Design review of the part built by this model. Coordinates are the model's own, in mm. A direction names the side the tool comes from. Round coordinates to 2 decimals unless told otherwise and drop trailing zeros. Write each loop counter-clockwise with the first axis right and the second up, starting at its lowest first coordinate (ties: lowest second). Pieces come first, ordered by that corner, then holes. Notation, with made-up numbers: (71, -34.75) - (123, -34.75) arc R20 cw to (123, -27.75) - close; hole circle Ø10 at (37, 70). An arc over 180 degrees is marked (long way). Use one line per item in the form item = value.
```python
from build123d import *

# Parameters (mm, degrees)
SKETCH1_W               = 26
SKETCH1_H               = 40
BOSS_EXTRUDE1_DEPTH     = 32
SKETCH2_W               = 21
SKETCH2_H               = 34.5
CUT_EXTRUDE1_DEPTH      = 28
SKETCH3_W               = 26
SKETCH3_H               = 25.26
BOSS_EXTRUDE2_DEPTH     = 20
SKETCH4_W               = 22
SKETCH4_H               = 19.76
CUT_EXTRUDE2_DEPTH      = 20
SKETCH5_W               = 21
SKETCH5_H               = 2.75
CUT_EXTRUDE3_DEPTH      = 25
SKETCH6_R               = 1.1
CUT_EXTRUDE4_DEPTH      = 20
SKETCH7_R               = 4
CUT_EXTRUDE5_DEPTH      = 5
SKETCH9_W               = 26
SKETCH9_H               = 25.26
CUT_EXTRUDE9_DEPTH      = 3
SKETCH10_R              = 4.8
SKETCH10_R_2            = 4
BOSS_EXTRUDE3_DEPTH     = 3
CUT_EXTRUDE10_DEPTH     = 5
SKETCH14_W              = 1.5
SKETCH14_H              = 19.76
BOSS_EXTRUDE5_DEPTH     = 17
SKETCH8_R               = 1
SKETCH8_R_2             = 1.3
CUT_EXTRUDE8_DEPTH      = 17
CUT_EXTRUDE8_DEPTH_BACK = 15
SKETCH17_W              = 26
SKETCH17_H              = 25.26
SKETCH17_W_2            = 20.5
SKETCH17_H_2            = 19.76
BOSS_EXTRUDE12_DEPTH    = 12
SKETCH18_W              = 21
SKETCH18_H              = 12
CUT_EXTRUDE11_DEPTH     = 5


with BuildPart() as part:
    # Sketch1 → Boss-Extrude1 (new body)
    with BuildSketch(Plane.XY):
        with Locations((-13, 20)):
            Rectangle(SKETCH1_W, SKETCH1_H)
    extrude(amount=BOSS_EXTRUDE1_DEPTH)

    # Sketch2 → Cut-Extrude1 (cut)
    with BuildSketch(Plane.XY.offset(32)):
        with Locations((-13, 20)):
            Rectangle(SKETCH2_W, SKETCH2_H)
    extrude(amount=-CUT_EXTRUDE1_DEPTH, mode=Mode.SUBTRACT)

    # Sketch3 → Boss-Extrude2 (add)
    with BuildSketch(Plane.XY.offset(32)):
        with Locations((-13, 12.63)):
            Rectangle(SKETCH3_W, SKETCH3_H)
    extrude(amount=BOSS_EXTRUDE2_DEPTH)

    # Sketch4 → Cut-Extrude2 (cut)
    with BuildSketch(Plane.XY.offset(52)):
        with Locations((-13, 12.63)):
            Rectangle(SKETCH4_W, SKETCH4_H)
    extrude(amount=-CUT_EXTRUDE2_DEPTH, mode=Mode.SUBTRACT)

    # Sketch5 → Cut-Extrude3 (cut)
    with BuildSketch(Plane.XY.offset(32)):
        with Locations((-13, 38.625)):
            Rectangle(SKETCH5_W, SKETCH5_H)
    extrude(amount=-CUT_EXTRUDE3_DEPTH, mode=Mode.SUBTRACT)

    # Sketch6 → Cut-Extrude4 (cut)
    with BuildSketch(Plane(origin=(0, 0, 0), x_dir=(-1, 0, 0), z_dir=(0, 0, -1))):
        with Locations((4.8, 4.55)):
            Circle(SKETCH6_R)
        with Locations((20.8, 4.55)):
            Circle(SKETCH6_R)
        with Locations((20.8, 34.55)):
            Circle(SKETCH6_R)
        with Locations((4.8, 34.55)):
            Circle(SKETCH6_R)
    extrude(amount=-CUT_EXTRUDE4_DEPTH, mode=Mode.SUBTRACT)

    # Sketch7 → Cut-Extrude5 (cut)
    with BuildSketch(Plane.ZY.offset(26)):
        with Locations((40, 12.51)):
            Circle(SKETCH7_R)
    extrude(amount=-CUT_EXTRUDE5_DEPTH, mode=Mode.SUBTRACT)

    # Sketch9 → Cut-Extrude9 (cut)
    with BuildSketch(Plane.XY.offset(52)):
        with Locations((-13, 12.63)):
            Rectangle(SKETCH9_W, SKETCH9_H)
    extrude(amount=-CUT_EXTRUDE9_DEPTH, mode=Mode.SUBTRACT)

    # Sketch10 → Boss-Extrude3 (add)
    with BuildSketch(Plane.ZY.offset(26)):
        with Locations((40, 12.51)):
            Circle(SKETCH10_R)
        with Locations((40, 12.51)):
            Circle(SKETCH10_R_2, mode=Mode.SUBTRACT)
    extrude(amount=BOSS_EXTRUDE3_DEPTH)

    # Sketch13 → Cut-Extrude10 (cut, through all)
    with BuildSketch(Plane.XY.offset(4)):
        Polygon((-23.5, 20), (-23.5, 12), (-2.5, 12), (-2.5, 29), (-23.5, 29), align=None)
    extrude(amount=-CUT_EXTRUDE10_DEPTH, mode=Mode.SUBTRACT)

    # Sketch14 → Boss-Extrude5 (add)
    with BuildSketch(Plane.XY.offset(49)):
        with Locations((-2.75, 12.63)):
            Rectangle(SKETCH14_W, SKETCH14_H)
    extrude(amount=-BOSS_EXTRUDE5_DEPTH)

    # Sketch8 → Cut-Extrude8 (cut, two sides)
    with BuildSketch(Plane(origin=(0, 0, 0), x_dir=(0, 0, -1), z_dir=(1, 0, 0))) as cut_extrude8_sk:
        with Locations((-40, 12.51)):
            Circle(SKETCH8_R)
        with Locations((-46, 12.51)):
            Circle(SKETCH8_R_2)
        with Locations((-34, 12.51)):
            Circle(SKETCH8_R_2)
        with Locations((-40, 18.51)):
            Circle(SKETCH8_R_2)
        with Locations((-40, 6.51)):
            Circle(SKETCH8_R_2)
    extrude(amount=CUT_EXTRUDE8_DEPTH, mode=Mode.SUBTRACT)
    extrude(cut_extrude8_sk.sketch, amount=-CUT_EXTRUDE8_DEPTH_BACK, mode=Mode.SUBTRACT)

    # Sketch17 → Boss-Extrude12 (add)
    with BuildSketch(Plane.XY.offset(49)):
        with Locations((-13, 12.63)):
            Rectangle(SKETCH17_W, SKETCH17_H)
        with Locations((-13.75, 12.63)):
            Rectangle(SKETCH17_W_2, SKETCH17_H_2, mode=Mode.SUBTRACT)
    extrude(amount=BOSS_EXTRUDE12_DEPTH)

    # Sketch18 → Cut-Extrude11 (cut)
    with BuildSketch(Plane(origin=(0, 25.26, 0), x_dir=(1, 0, 0), z_dir=(0, 1, 0))):
        with Locations((-13, -38)):
            Rectangle(SKETCH18_W, SKETCH18_H)
    extrude(amount=-CUT_EXTRUDE11_DEPTH, mode=Mode.SUBTRACT)


solid = part.part
```
Q1. Machinability: for faces 4 (the flat face through (0, 15, 30)), 5 (the flat face through (-1, 33, 32)), 6 (the cylindrical face through (-1.73, 6.57, 41.3)), 7 (the flat face through (-13, 33, 4)), 8 (the flat face through (-13, 40, 5)), which of the approach directions +Z, -Z, +X, -X, +Y, -Y give a long, thin tool a straight path to every point of the face, cutting with its end or side? Answer none if there is none.
Calculated:
face_4 = +Z, -Z, +X, +Y, -Y
face_5 = +Z, +X, -X, +Y
face_6 = +X
face_7 = +Z
face_8 = +Z, -Z, +X, -X, +Y
Q2. We need section C-C on x = -9. Write out the cut boundary in (y, z).
Calculated:
outline = (0, 0) - (12, 0) - (12, 4) - (2.75, 4) - (2.75, 61) - (0, 61) - close; (22.51, 44) - (25.26, 44) - (25.26, 61) - (22.51, 61) - close; (29, 0) - (40, 0) - (40, 7) - (37.25, 7) - (37.25, 4) - (29, 4) - close
Q3. For P1, Ø5, axis at x = -25.5, z = 27, coming from the -Y side; P2, Ø9, axis at x = -12.5, y = 34.5, coming from the +Z side; P3, Ø2.5, axis at y = 12.51, z = 40, coming from the -X side; P4, Ø3, axis at x = -19, y = 4.5, coming from the +Z side, all flat-tipped, find the tip position at first contact; note any pin that passes through.
Calculated:
P1 = 0
P2 = 7
P3 = -3.5
P4 = 4
Q4. To check wall thickness, follow line 1 along Y through (x, z) = (-20.8, 1); line 2 along X through (y, z) = (5, 20.5); line 3 along X through (y, z) = (15, 45). State the ranges of each line that lie inside material, in increasing order. Write a range as from..to.
Calculated:
line_1 = 0..3.45, 5.65..12, 29..33.45, 35.65..40
line_2 = -26..-23.5, -2.5..0
line_3 = -26..-24, -3.5..0
Q5. We need section A-A on y = 34.55. Write out the cut boundary in (x, z), then the cut area to 3 significant figures.
Calculated:
outline = (-26, 0) - (-21.9, 0) - (-21.9, 4) - (-23.5, 4) - (-23.5, 32) - (-26, 32) - close; (-19.7, 0) - (-5.9, 0) - (-5.9, 4) - (-19.7, 4) - close; (-3.7, 0) - (0, 0) - (0, 32) - (-2.5, 32) - (-2.5, 4) - (-3.7, 4) - close
area = 226 mm2
Q6. We need section D-D on y = 6.51. Write out the cut boundary in (x, z).
Calculated:
outline = (-26, 0) - (0, 0) - (0, 38.7) - (-3.5, 38.7) - (-3.5, 32) - (-2.5, 32) - (-2.5, 4) - (-23.5, 4) - (-23.5, 32) - (-24, 32) - (-24, 61) - (-26, 61) - close; (-3.5, 41.3) - (0, 41.3) - (0, 61) - (-3.5, 61) - close
Q7. We need section B-B on x = -20.8. Write out the cut boundary in (y, z), then the cut area to 3 significant figures.
Calculated:
outline = (0, 0) - (3.45, 0) - (3.45, 4) - (2.75, 4) - (2.75, 61) - (0, 61) - close; (5.65, 0) - (12, 0) - (12, 4) - (5.65, 4) - close; (22.51, 44) - (25.26, 44) - (25.26, 61) - (22.51, 61) - close; (29, 0) - (33.45, 0) - (33.45, 4) - (29, 4) - close; (35.65, 0) - (40, 0) - (40, 7) - (37.25, 7) - (37.25, 4) - (35.65, 4) - close
area = 286 mm2
Q8. Draft analysis for pull direction Y (two halves, no side actions). For faces 1 (the flat face through (-13, 39, 7)), 2 (the flat face through (-13, 7, 4)), 3 (the cylindrical face through (-27.479, 7.824, 38.959)), state which applies: released by +Y, released by -Y, zero draft, split by the parting line, or undercut.
Calculated:
face_1 = zero draft
face_2 = undercut
face_3 = split by the parting line
